```python
from build123d import *

# Parameters (mm, degrees)
BOSS_EXTRUDE1_DEPTH      = 0.5
BOSS_EXTRUDE2_DEPTH      = 12
BOSS_EXTRUDE2_DEPTH_BACK = 0.6
SKETCH2_R                = 1
FILLET1_R                = 1
SKETCH3_R                = 0.8
CUT_EXTRUDE1_DEPTH       = 0.5
FILLET2_R                = 0.1


with BuildPart() as part:
    # Sketch1 → Boss-Extrude1 (new body)
    with BuildSketch(Plane(origin=(0, 0, 0), x_dir=(0, 0, -1), z_dir=(1, 0, 0))):
        with BuildLine():
            Line((0, 0), (0, 7.177124344))
            ThreePointArc((0, 7.177124344), (-0.5, 8.5), (0, 9.822875656))
            Line((0, 9.822875656), (3, 9.822875656))
            ThreePointArc((3, 9.822875656), (3.5, 8.5), (3, 7.177124344))
            Line((3, 7.177124344), (3, 0))
            ThreePointArc((3, 0), (1.5, -1.5), (0, 0))
        make_face()
    extrude(amount=BOSS_EXTRUDE1_DEPTH)

    # Sketch2 → Boss-Extrude2 (add, two sides: drawn at the far end of the back side and taken through both)
    with BuildSketch(Plane(origin=(0.5, 0, 0), x_dir=(0, 0, -1), z_dir=(1, 0, 0)).offset(-BOSS_EXTRUDE2_DEPTH_BACK)):
        with Locations((1.5, 8.5)):
            Circle(SKETCH2_R)
    extrude(amount=BOSS_EXTRUDE2_DEPTH + BOSS_EXTRUDE2_DEPTH_BACK)

    # Fillet1
    fillet1_edges = [part.edges().sort_by_distance(p)[0] for p in [
        (12.5, 8.5, -0.5),
    ]]
    fillet(fillet1_edges, radius=FILLET1_R)

    # Sketch3 → Cut-Extrude1 (cut)
    with BuildSketch(Plane.ZY.offset(0.1)):
        with Locations((-1.5, 8.5)):
            Circle(SKETCH3_R)
    extrude(amount=-CUT_EXTRUDE1_DEPTH, mode=Mode.SUBTRACT)

    # Fillet2
    fillet2_edges = [part.edges().sort_by_distance(p)[0] for p in [
        (-0.1, 8.5, -0.5),
        (0.4, 8.5, -2.3),
        (-0.1, 8.5, -2.3),
    ]]
    fillet(fillet2_edges, radius=FILLET2_R - 0.0001)  # a hair under: the kernel refuses the full size


solid = part.part
```
Input: part model. Units: mm. Frame: model coordinates. A direction names the side the tool comes from. Give positions to 0.01 mm unless a question says otherwise; leave off trailing zeros. Loops run counter-clockwise (first coordinate to the right, second up) from the corner with the lowest first, then second, coordinate; pieces in that order, holes last.
1) Line query: L1, parallel to Y at x = 0.2, z = -1.5; L2, parallel to X at y = 9, z = -2.7; L3, parallel to Y at x = 3.5, z = -1.45. Output: solid intervals per line, ascending.
A:
L1: y = -1.5 to 7.7, 9.3 to 9.82
L2: x = 0 to 0.5
L3: y = 7.5 to 9.5
2) Section query D-D on y = 4.25. Return the cut outline in (x, z).
A:
outline: (0, -3) - (0.5, -3) - (0.5, 0) - (0, 0) - close
3) Reachability of faces 4 (the cylindrical face through (0.15, 9.04, -2.09)), 5 (the cylindrical face through (0.2, -1.5, -1.5)) from +Z, -Z, +X, -X, +Y, -Y: full face, straight path, thin tool, end or side. Return the list, or none.
A:
face 4: -X
face 5: +X, -X, -Y
4) Contact query for a flat-ended pin moving along its axis: pin 1 (1.3 mm diameter, centred on y = 8.5, z = -1.5, fed in from -X). Output: stop coordinate, or through.
A:
pin 1: stops at x = 0.4
5) Section query C-C on x = 4.75. Return the cut outline in (y, z), and give its area (3 significant figures).
A:
outline: circle Ø2 at (8.5, -1.5)
area: 3.14 mm2
6) Mould query, pull axis Z, two halves, no side actions, for faces 1 (the flat face through (0, 4, -2)), 2 (the flat face through (0.4, 8.5, -1.5)), 3 (the cylindrical face through (5.92, 9.49, -1.37)). Classes: released by +Z, released by -Z, zero draft, split by the parting line, or undercut.
A:
face 1: zero draft
face 2: undercut
face 3: split by the parting line
